Geometry: final body of the model. Coordinates: model frame, mm. A direction names the side the tool comes from. Give positions to 0.01 mm unless a question says otherwise; leave off trailing zeros. Write each loop counter-clockwise with the first axis right and the second up, starting at its lowest first coordinate (ties: lowest second). Pieces come first, ordered by that corner, then holes. Notation, with made-up numbers: (-15, 85) -> (25, 85) arc R13 ccw to (25, 93) -> close; hole circle Ø11 at (84.5, 55.25). An arc over 180 degrees is marked (long way). Use CSV: the item, a comma, the result in double quotes. Start each with the question number.
1) Section B-B (x = 0.75). Output: boundary loops of the cut face in (y, z), plus the area to 3 significant figures.
2) Set-up query: faces 1 (the face through (8.37, -1.5, -0.07)), 2 (the face through (-0.159, -0.596, 2.685)), 3 (the face through (-1.5, -0.4, 0)). Return all of +Z, -Z, +X, -X, +Y, -Y with unobstructed straight access to the full face (end or side cutting, diameter ignored); none if empty.
3) Contact query for flat-ended pins moving along their axis: P1, Ø1.3, axis at x = -1.5, z = 1.5, coming from the +Y side; P2, Ø1.5, axis at x = 2, y = 0, coming from the +Z side; P3, Ø0.6, axis at x = -2, z = -1, coming from the -Y side. Output: stop coordinate, or through.
4) Section A-A (x = 13). Output: boundary loops of the cut face in (y, z), plus the area to 3 significant figures.
5) Material intervals for line 1 (X direction, y = -0.5, z = 0.2); line 2 (X direction, y = 0, z = -1.6); line 3 (Y direction, x = 1.25, z = 0.5), sorted ascending. Write a range as [from, to].
6) Draft query along X for faces 4 (the face through (0.465, 1.244, 0.516)), 5 (the face through (16, 0, 0)), 6 (the face through (-1.5, 0.4, 0)), 7 (the face through (-0.939, 0, 0)). Return one class per face: pulls with the +X half, pulls with the -X half, needs draft (parallel to the pull), parting line crosses it, or undercut.
Autodesk Inventor part; units mm, degrees
ref_plane "IDS_WORKPLANE{1}" through (-2.1389, 0, 0) normal (1, 0, 0) x (0, 0, -1)
ref_plane "Work Plane2" through (8.25, 0, 0) normal (0, 0, -1) x (1, 0, 0)
ref_plane "YZ Plane" through (0, 0, 0) normal (1, 0, 0) x (0, 1, 0)
sketch "Skizze1" plane through (0, 0, 0) normal (0, 0, 1) x (1, 0, 0)
  line L0 (-2.1389, 0) -> (16, 0)
  line L1 (16, 0) -> (16, 1.5)
  line L2 (16, 1.5) -> (1.25, 1.5)
  line L3 (1.25, 1.5) -> (0.9433, 1.3468)
  line L4 (0.9433, 1.3468) -> (0, 1.3467)
  line L5 (0, 1.3467) -> (0, 2.75)
  line L6 (-6.0203, 0) -> (20.8022, 0)
  line L7 (0, -0.5507) -> (0, 3.3039)
  line L8 (0, 2.75) -> (-1.94, 2.7497)
  arc A0 (-1.94, 2.7497) -> (-2.1389, 0) centre (16.9704, 0) ccw
  dimension "d0" = 16
  dimension "d1" = 14.75
  dimension "d2" = 0.3067
  dimension "d3" = 2.1389
  dimension "d4" = 3
  dimension "d5" = 2.6935
  dimension "d9" = 5.5
  dimension "d10" = 0.01
  dimension "d15" = 19.1093
revolve "Körper" add sketch "Skizze1" angle 360 about axis through (-2.1389, 0, 0) along (1, 0, 0)
fillet "Rundung1" radius 1.8 1 edges at (-1.94, -2.7497, 0)
ref_plane "IDS_WORKPLANE{1}" through (-2.1389, 0, 0) normal (1, 0, 0) x (0, 0, -1)
sketch "Skizze2" plane through (-2.1389, 0, 0) normal (1, 0, 0) x (0, 0, -1)
  line L0 (0, -3.85) -> (0, 3.85)
  line L1 (3.85, 0) -> (-3.85, 0)
  line L2 (-2.75, 0.4) -> (2.75, 0.4)
  line L3 (2.75, 0.4) -> (2.75, -0.4)
  line L4 (2.75, -0.4) -> (-2.75, -0.4)
  line L5 (-2.75, -0.4) -> (-2.75, 0.4)
  line L6 (0, 0.4) -> (0, -0.4) construction
  line L7 (-2.75, 0) -> (2.75, 0) construction
  circle A0 centre (0, 0) radius 2.75
  dimension "d17" = 0.8
extrude "Loch" cut sketch "Skizze2" along normal blind 1.2 contours L4 A0 L1 L0 | L0 L1 A0 L4 | L4 L5 A0 | A0 L3 L4 | L1 A0 L2 L0 | L0 L2 A0 L1 | L5 L2 A0 | A0 L2 L3
thread "Gewinde"
chamfer "Fase1" distance 0.3067 distance2 0.3068 1 edges at (16, -1.5, 0) measured on face at (16, 0.481, 0.3876)
ref_plane "Work Plane2" through (8.25, 0, 0) normal (0, 0, -1) x (1, 0, 0)
equation "\"d0\" = NLG"
equation "\"d1\" = GEL"
equation "\"d2\" = GAL"
equation "\"d3\" = KOH"
equation "\"d4\" = GD"
equation "\"d5\" = BDM"
equation "\"d9\" = KOD"
equation "\"d10\" = KEWI"
equation "\"d17\" = SBR"
equation "\"d18\" = STI"
equation "\"d20\" = RR"
equation "\"d11\" = GEL"
equation "\"d13\" = -0.5 * SPD + 0.5 * GD"
equation "\"GD\" = NND"
equation "\"NLG\" = 16"
equation "\"GEL\" = 14.75"
equation "\"KOD\" = 5.5"
equation "\"KOH\" = 2.13889"
equation "\"GAL\" = 0.61345 * PTC"
equation "\"SPD\" = NND - 1.2269 * PTC"
equation "\"BDM\" = 2.6935"
equation "\"GUL\" = 0.61345 * PTC"
equation "\"RR\" = 1.8"
equation "\"SBR\" = 0.8"
equation "\"STI\" = 1.2"
equation "\"KEWI\" = 0.01deg"
equation "\"KR\" = 3.3"
equation "\"d16\" = -KOH"
equation "\"PTC\" = 0.5"
equation "\"THREADDIA\" = 3"
equation "\"TOA\" = 30deg"
equation "\"NND\" = 3"
equation "\"ORI\" = 1.8"
equation "\"GD1\" = THREADDIA - 1.2269 * PTC"
properties part number "CNS 9671 - M3 x 16" material "Steel, Mild"
Answers follow:
1,outline,"circle Ø2.69 at (0, 0)"
1,area,"5.70 mm^2"
2,face 1,"+X"
2,face 2,"+X, -X"
2,face 3,"+Z, -Z, -X"
3,P1,"stops at y = 2.38"
3,P2,"stops at z = 1.5"
3,P3,"stops at y = -1.87"
4,outline,"circle Ø3 at (0, 0)"
4,area,"7.07 mm^2"
5,line 1,"x = [-2.13, 16]"
5,line 2,"x = [-0.94, 0]"
5,line 3,"y = [-1.41, 1.41]"
6,face 4,"undercut"
6,face 5,"pulls with the +X half"
6,face 6,"needs draft"
6,face 7,"pulls with the -X half"
